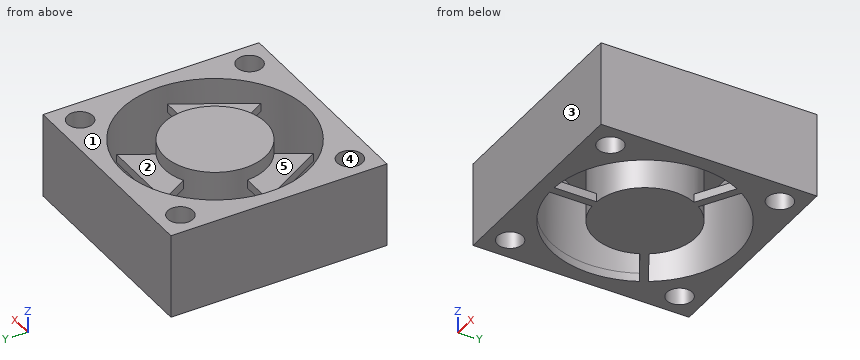
Autodesk Inventor part; units mm, degrees
ref_plane "Work Plane1" through (0, 0, 8.4) normal (0, 0, 1) x (1, 0, 0)
ref_plane "YZ Plane" through (0, 0, 0) normal (1, 0, 0) x (0, 1, 0)
ref_plane "XZ Plane" through (0, 0, 0) normal (0, 1, 0) x (-1, 0, 0)
sketch "Sketch1" plane through (0, 0, 0) normal (0, 0, 1) x (1, 0, 0)
  line L0 (0, -17.85) -> (0, 17.85) construction
  line L1 (-17.85, 0) -> (17.85, 0) construction
  line L2 (-12.75, 12.75) -> (12.75, 12.75)
  line L3 (12.75, 12.75) -> (12.75, -12.75)
  line L4 (12.75, -12.75) -> (-12.75, -12.75)
  line L5 (-12.75, -12.75) -> (-12.75, 12.75)
  line L6 (-12.75, 12.75) -> (12.75, -12.75) construction
  line L7 (12.75, 12.75) -> (-12.75, -12.75) construction
  circle A0 centre (-10, -10) radius 1.5
  circle A1 centre (10, -10) radius 1.5
  circle A2 centre (-10, 10) radius 1.5
  circle A3 centre (10, 10) radius 1.5
  circle A4 centre (0, 0) radius 6
  circle A5 centre (0, 0) radius 11
  dimension "d0" = 25.5
  dimension "d1" = 25.5
  dimension "d2" = 3
  dimension "d3" = 3
  dimension "d4" = 20
  dimension "d5" = 2.75
  dimension "d7" = 2.75
  dimension "d8" = 2.75
  dimension "d9" = 12
  dimension "d10" = 22
extrude "Extrusion1" add sketch "Sketch1" along normal blind 10
extrude "Extrusion2" add sketch "Sketch1" along normal blind 1 contours A5
sketch "Sketch3" plane through (0, 0, 0) normal (0, 0, -1) x (-1, 0, 0)
  circle A0 centre (0, 0) radius 6
  line L0 (-5.4158, 2.5824) -> (-9.7489, 5.095)
  circle A1 centre (0, 0) radius 11
  line L1 (-4.9551, 3.3833) -> (-9.2869, 5.8953)
  line L2 (0.4715, -5.9814) -> (0.462, -10.9903)
  line L3 (-0.4525, -5.9829) -> (-0.462, -10.9903)
  line L4 (4.9443, 3.399) -> (9.2869, 5.8953)
  line L5 (5.4076, 2.5996) -> (9.7489, 5.095)
  dimension "d17" = 0.924
  dimension "d18" = 0.924
  dimension "d21" = 360
  dimension "d23" = 120
  dimension "d24" = 0.924
extrude "Extrusion3" cut sketch "Sketch3" against normal blind 1 contours A0 L5 A1 L2 | A0 L1 A1 L4 | L3 A1 L0 A0
ref_plane "Work Plane1" through (0, 0, 8.4) normal (0, 0, 1) x (1, 0, 0)
sketch "Sketch4" plane through (0, 0, 8.4) normal (0, 0, 1) x (1, 0, 0)
  circle A0 centre (0, 0) radius 6
  line L0 (-2.75, 5.3327) -> (-4.75, 8.7968)
  line L1 (-4.75, 8.7968) -> (4.75, 8.7968)
  line L2 (4.75, 8.7968) -> (2.75, 5.3327)
  line L3 (-12.75, 12.75) -> (-12.75, -12.75)
  line L4 (12.75, -12.75) -> (12.75, 12.75)
  line L5 (-3.2432, -5.0479) -> (-5.2432, -8.512)
  line L6 (-5.2432, -8.512) -> (-9.9932, -0.2848)
  line L7 (-9.9932, -0.2848) -> (-5.9932, -0.2848)
  line L8 (5.9932, -0.2848) -> (9.9932, -0.2848)
  line L9 (9.9932, -0.2848) -> (5.2432, -8.512)
  line L10 (5.2432, -8.512) -> (3.2432, -5.0479)
  dimension "d28" = 8
  dimension "d29" = 8
  dimension "d30" = 10
  dimension "d31" = 60
  dimension "d32" = 60
  dimension "d35" = 360
extrude "Extrusion4" add sketch "Sketch4" against normal blind 1 contours A0 L0 L1 L2 | L8 L9 L10 A0 | A0 L5 L6 L7
properties part number "maly_wentylator"
The listing builds one solid part. Answer for the finished solid, in the listing's coordinates (mm). Face numbers are marked on the shaded views. A direction names the side the tool comes from. Coordinates: 2 decimals unless noted, no trailing zeros. Order: outer loops, then holes, each group sorted by start corner. A loop starts at its lowest first (then second) coordinate and runs counter-clockwise, first axis right, second up.
Q1. Given P1, Ø1, axis at x = 0, y = -8, coming from the +Z side; P2, Ø3, axis at x = 0.5, y = 8, coming from the +Z side; P3, Ø2, axis at x = -7, y = -5, coming from the -Z side, each flat-ended and moving along its own axis, determine where each tip first touches the part or whether it passes through.
Q2. A cutting plane is placed at A-A, the plane y = -8. Write down the section's boundary in (x, z), and give its area (3 significant figures).
Q3. Consider line 1 (Y direction, x = 0, z = 5); line 2 (Y direction, x = 10, z = 7.25); line 3 (Y direction, x = -9, z = 7.5). Determine where each line is inside the solid, lowest interval first.
Q4. A cutting plane is placed at D-D, the plane x = -7.5. Write down the section's boundary in (y, z).
Q5. For a pull along Y with two mould halves and no side action, classify the marked faces 1, 2 and 3 as pulls with the +Y half, pulls with the -Y half, needs draft (parallel to the pull), parting line crosses it, or undercut.
Q6. A cutting plane is placed at C-C, the plane z = 4.25. Write down the section's boundary in (x, y), and give its area (3 significant figures).
Q7. Which of the six approach directions +Z, -Z, +X, -X, +Y, -Y give full straight-line access (tool end or side, diameter ignored) to the marked faces 4 and 5?
Answers follow:
1. P1: stops at z = 1
1. P2: stops at z = 8.4
1. P3: stops at z = 7.4
2. outline: (-12.75, 0) - (-7.55, 0) - (-7.55, 10) - (-12.75, 10) - close; (-5.54, 7.4) - (-4.95, 7.4) - (-4.95, 8.4) - (-5.54, 8.4) - close; (-0.47, 0) - (0.46, 0) - (0.46, 1) - (-0.47, 1) - close; (4.95, 7.4) - (5.54, 7.4) - (5.54, 8.4) - (4.95, 8.4) - close; (7.55, 0) - (12.75, 0) - (12.75, 10) - (7.55, 10) - close
2. area: 106 mm2
3. line 1: y = -12.75 to -11, -6 to 6, 11 to 12.75
3. line 2: y = -12.75 to -11.5, -8.5 to -4.58, 4.58 to 8.5, 11.5 to 12.75
3. line 3: y = -12.75 to -11.12, -8.88 to -6.32, -2.01 to -0.28, 6.32 to 8.88, 11.12 to 12.75
4. outline: (-12.75, 0) - (-8.05, 0) - (-8.05, 10) - (-12.75, 10) - close; (-4.6, 7.4) - (-0.28, 7.4) - (-0.28, 8.4) - (-4.6, 8.4) - close; (3.8, 0) - (4.87, 0) - (4.87, 1) - (3.8, 1) - close; (8.05, 0) - (12.75, 0) - (12.75, 10) - (8.05, 10) - close
5. face 1: needs draft
5. face 2: undercut
5. face 3: pulls with the -Y half
6. outline: (-12.75, -12.75) - (12.75, -12.75) - (12.75, 12.75) - (-12.75, 12.75) - close; circle Ø12 at (0, 0); hole circle Ø3 at (-10, -10); hole circle Ø3 at (-10, 10); hole circle Ø22 at (0, 0); hole circle Ø3 at (10, -10); hole circle Ø3 at (10, 10)
6. area: 355 mm2
7. face 4: +Z, -Z
7. face 5: +Z
